from build123d import *

# Parameters (mm, degrees)
F1_DEPTH = 10.16


with BuildPart() as f1:
    # F0 (on Front) → F1 (new body)
    with BuildSketch(Plane.XZ):
        with BuildLine():
            Line((0, 60.325), (0, 0))
            Line((0, 0), (215.9, 0))
            Line((215.9, 0), (215.9, 177.8))
            Line((215.9, 177.8), (15.875, 177.8))
            Line((15.875, 177.8), (15.875, 76.2))
            ThreePointArc((15.875, 76.2), (11.22532, 64.97468), (0, 60.325))
        make_face()
    extrude(amount=F1_DEPTH)

    # F2: F1 across plane


with BuildPart() as f1_1:
    add(f1.part)
    add(f1.part.mirror(Plane.YZ))


solid = f1_1.part
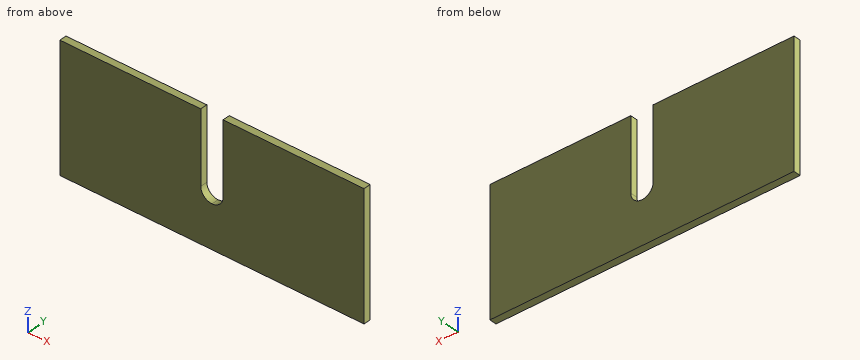
The listing builds one solid part. Answer for the finished solid, in the listing's coordinates (mm). Give positions to 0.01 mm unless a question says otherwise; leave off trailing zeros. Write each loop counter-clockwise with the first axis right and the second up, starting at its lowest first coordinate (ties: lowest second). Pieces come first, ordered by that corner, then holes. Notation, with made-up numbers: (36, 58) - (50, 58) arc R28 cw to (50, 87) - close; hole circle Ø11 at (-29, 24.5). An arc over 180 degrees is marked (long way). Use a Markdown table: item, result.
1. Section B-B on y = -5 is taken. Write down the section's boundary in (x, z) (3 decimals), plus the area to 3 significant figures.
Values follow:
| item | result |
|---|---|
| outline | (-215.9, 0) - (215.9, 0) - (215.9, 177.8) - (15.875, 177.8) - (15.875, 76.2) arc R15.875 cw to (0, 60.325) arc R15.875 cw to (-15.875, 76.2) - (-15.875, 177.8) - (-215.9, 177.8) - close |
| area | 73,200 mm² |
2. Find the intervals of material crossed by probe 1 along X at (y, z) = (-6.5, 118.5) (3 decimals), in increasing order. Write a range as from..to.
Values follow:
| item | result |
|---|---|
| probe 1 | x = -215.9..-15.875, 15.875..215.9 |
3. Section A-A on z = 156 is taken. Write down the section's boundary in (x, y) (3 decimals), plus the area to 3 significant figures.
Values follow:
| item | result |
|---|---|
| outline | (-215.9, -10.16) - (-15.875, -10.16) - (-15.875, 0) - (-215.9, 0) - close; (15.875, -10.16) - (215.9, -10.16) - (215.9, 0) - (15.875, 0) - close |
| area | 4,060 mm² |
4. This flat-tipped pin is pushed along its axis until it touches: P1, Ø5, axis at x = -68, y = -1.5, coming from the -Z side. Where does it stop, or does it pass through?
Values follow:
| item | result |
|---|---|
| P1 | stops at z = 0 |
